Geometry: final body of the model. Coordinates: model frame, mm. Face numbers are marked on the shaded views. A direction names the side the tool comes from. Give positions to 0.01 mm unless a question says otherwise; leave off trailing zeros. Order: outer loops, then holes, each group sorted by start corner. A loop starts at its lowest first (then second) coordinate and runs counter-clockwise, first axis right, second up. Notation, with made-up numbers: (75.25, -31) - (98.25, -31) arc R9 ccw to (98.25, -27) - close; hole circle Ø6 at (77.5, -18). An arc over 180 degrees is marked (long way). One line per item, written item: value.
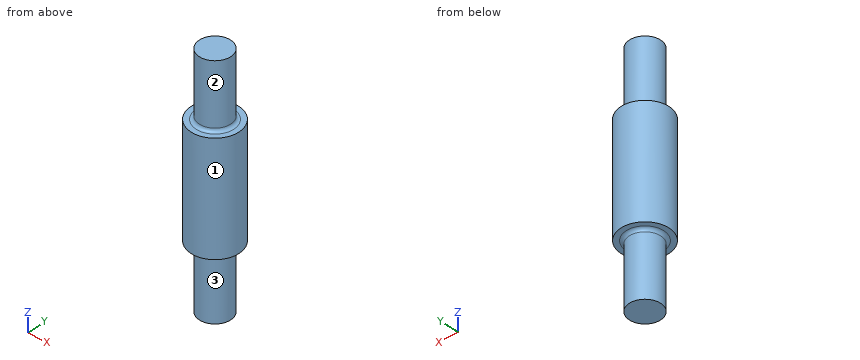
```python
from build123d import *

# Parameters (mm, degrees)
SKETCH2_R           = 13
BOSS_EXTRUDE1_DEPTH = 130
SKETCH3_R           = 13
SKETCH3_R_2         = 8.5
CUT_EXTRUDE1_DEPTH  = 35
SKETCH4_R           = 13
SKETCH4_R_2         = 8.5
CUT_EXTRUDE2_DEPTH  = 35
FILLET1_R           = 1.7
FILLET2_R           = 1.7


with BuildPart() as part:
    # Sketch2 → Boss-Extrude1 (new body)
    with BuildSketch(Plane.XY):
        Circle(SKETCH2_R)
    extrude(amount=BOSS_EXTRUDE1_DEPTH)

    # Sketch3 → Cut-Extrude1 (cut)
    with BuildSketch(Plane.XY.offset(130)):
        Circle(SKETCH3_R)
        Circle(SKETCH3_R_2, mode=Mode.SUBTRACT)
    extrude(amount=-CUT_EXTRUDE1_DEPTH, mode=Mode.SUBTRACT)

    # Sketch4 → Cut-Extrude2 (cut)
    with BuildSketch(Plane(origin=(0, 0, 0), x_dir=(-1, 0, 0), z_dir=(0, 0, -1))):
        Circle(SKETCH4_R)
        Circle(SKETCH4_R_2, mode=Mode.SUBTRACT)
    extrude(amount=-CUT_EXTRUDE2_DEPTH, mode=Mode.SUBTRACT)

    # Fillet1
    fillet1_edges = [part.edges().sort_by_distance(p)[0] for p in [
        (-8.5, 0, 95),
    ]]
    fillet(fillet1_edges, radius=FILLET1_R)

    # Fillet2
    fillet2_edges = [part.edges().sort_by_distance(p)[0] for p in [
        (8.5, 0, 35),
    ]]
    fillet(fillet2_edges, radius=FILLET2_R)


solid = part.part
```
1) Set-up query: the marked faces 1, 2 and 3. Return all of +Z, -Z, +X, -X, +Y, -Y with unobstructed straight access to the full face (end or side cutting, diameter ignored); none if empty.
Answers below:
face 1: +Z, -Z
face 2: +Z
face 3: -Z
2) First-contact query: pin 1 (5 mm diameter, centred on x = -5, z = 72, fed in from +Y); pin 2 (8 mm diameter, centred on y = -7.5, z = 90.5, fed in from +X); pin 3 (3 mm diameter, centred on y = 5.5, z = 21.5, fed in from -X); pin 4 (8 mm diameter, centred on x = 3.5, y = 8.5, fed in from +Z). Flat tips, straight axial feed; report the tip coordinate or a pass-through.
Answers below:
pin 1: y = 12.76
pin 2: x = 12.52
pin 3: x = -7.5
pin 4: z = 130
3) Material intervals for line 1 along Z through (x, y) = (9.75, -7.5); line 2 along Y through (x, z) = (8.5, 39); line 3 along Y through (x, z) = (2, 124), sorted ascending.
Answers below:
line 1: 35 to 95
line 2: -9.84 to 9.84
line 3: -8.26 to 8.26
4) Section C-C, the plane z = 112. Return loops of the section in (x, y), then the cut area to 3 significant figures.
Answers below:
outline: circle Ø17 at (0, 0)
area: 227 mm^2
5) Section A-A, the plane y = 0. Return loops of the section in (x, z).
Answers below:
outline: (-13, 35) - (-10.2, 35) arc R1.7 cw to (-8.5, 33.3) - (-8.5, 0) - (8.5, 0) - (8.5, 33.3) arc R1.7 cw to (10.2, 35) - (13, 35) - (13, 95) - (10.2, 95) arc R1.7 cw to (8.5, 96.7) - (8.5, 130) - (-8.5, 130) - (-8.5, 96.7) arc R1.7 cw to (-10.2, 95) - (-13, 95) - close
